from build123d import *

# Parameters (mm, degrees)
SKETCH1_R           = 5
BOSS_EXTRUDE1_DEPTH = 3
BOSS_EXTRUDE2_DEPTH = 3
BOSS_EXTRUDE3_DEPTH = 2.5
SKETCH4_R           = 3
CUT_EXTRUDE1_DEPTH  = 1
SKETCH5_R           = 1.25
CUT_EXTRUDE2_DEPTH  = 36.707142143
CUT_EXTRUDE3_DEPTH  = 3
SKETCH7_R           = 1
CUT_EXTRUDE4_DEPTH  = 36.860842154


with BuildPart() as part:
    # Sketch1 → Boss-Extrude1 (new body)
    with BuildSketch(Plane(origin=(0, 0, 0), x_dir=(1, 0, 0), z_dir=(0, 1, 0))):
        with Locations(Location((0, 0, 0), (0, 0, 270))):
            Circle(SKETCH1_R)
    extrude(amount=BOSS_EXTRUDE1_DEPTH)

    # Sketch2 → Boss-Extrude2 (add)
    with BuildSketch(Plane.XZ):
        with BuildLine():
            Line((-19, 6), (19, 6))
            ThreePointArc((19, 6), (25, 0), (19, -6))
            Line((19, -6), (-19, -6))
            ThreePointArc((-19, -6), (-25, 0), (-19, 6))
        make_face()
    extrude(amount=BOSS_EXTRUDE2_DEPTH)

    # Sketch3 → Boss-Extrude3 (add)
    with BuildSketch(Plane.XZ.offset(3)):
        with BuildLine():
            Line((-6, -19), (-6, 19))
            ThreePointArc((-6, 19), (0, 25), (6, 19))
            Line((6, 19), (6, -19))
            ThreePointArc((6, -19), (0, -25), (-6, -19))
        make_face()
    extrude(amount=-BOSS_EXTRUDE3_DEPTH)

    # Sketch4 → Cut-Extrude1 (cut)
    with BuildSketch(Plane.XZ.offset(3)):
        with Locations(Location((0, 0, 0), (0, 0, 270))):
            Circle(SKETCH4_R)
    extrude(amount=-CUT_EXTRUDE1_DEPTH, mode=Mode.SUBTRACT)

    # Sketch5 → Cut-Extrude2 (cut, through all)
    with BuildSketch(Plane.XZ.offset(2)):
        with Locations(Location((0, 0, 0), (0, 0, 270))):
            Circle(SKETCH5_R)
    extrude(amount=-CUT_EXTRUDE2_DEPTH, mode=Mode.SUBTRACT)

    # Sketch6 → Cut-Extrude3 (cut)
    with BuildSketch(Plane(origin=(0, 3, 0), x_dir=(1, 0, 0), z_dir=(0, 1, 0))):
        with BuildLine():
            Line((0.25, 2.25), (0.25, 1.984313483))
            ThreePointArc((0.25, 1.984313483), (0.367499036, 1.965946199), (0.483698652, 1.940627634))
            Line((0.483698652, 1.940627634), (0.579675692, 2.188372933))
            ThreePointArc((0.579675692, 2.188372933), (0.903104165, 2.331180574), (1.045911806, 2.0077521))
            Line((1.045911806, 2.0077521), (0.949934766, 1.760006801))
            ThreePointArc((0.949934766, 1.760006801), (1.052864326, 1.700434271), (1.15207112, 1.63484927))
            Line((1.15207112, 1.63484927), (1.331062969, 1.831193975))
            ThreePointArc((1.331062969, 1.831193975), (1.684239109, 1.847522293), (1.700567428, 1.494346153))
            Line((1.700567428, 1.494346153), (1.521575579, 1.298001448))
            ThreePointArc((1.521575579, 1.298001448), (1.596034455, 1.205269273), (1.66485, 1.108275452))
            Line((1.66485, 1.108275452), (1.902682817, 1.226702123))
            ThreePointArc((1.902682817, 1.226702123), (2.237908228, 1.114345889), (2.125551994, 0.779120478))
            Line((2.125551994, 0.779120478), (1.887719178, 0.660693807))
            ThreePointArc((1.887719178, 0.660693807), (1.923651286, 0.54732598), (1.952781662, 0.432022894))
            Line((1.952781662, 0.432022894), (2.217334807, 0.456537353))
            ThreePointArc((2.217334807, 0.456537353), (2.489335441, 0.230670899), (2.263468987, -0.041329735))
            Line((2.263468987, -0.041329735), (1.998915842, -0.065844194))
            ThreePointArc((1.998915842, -0.065844194), (1.991468353, -0.184536719), (1.97697934, -0.30257675))
            Line((1.97697934, -0.30257675), (2.232523445, -0.375285317))
            ThreePointArc((2.232523445, -0.375285317), (2.404564108, -0.684157475), (2.09569195, -0.856198138))
            Line((2.09569195, -0.856198138), (1.840147845, -0.783489572))
            ThreePointArc((1.840147845, -0.783489572), (1.790326583, -0.891476712), (1.734175003, -0.996311728))
            Line((1.734175003, -0.996311728), (1.94619742, -1.156423625))
            ThreePointArc((1.94619742, -1.156423625), (1.995043068, -1.506586591), (1.644880102, -1.555432239))
            Line((1.644880102, -1.555432239), (1.432857685, -1.395320341))
            ThreePointArc((1.432857685, -1.395320341), (1.347391287, -1.478017834), (1.257160723, -1.555489285))
            Line((1.257160723, -1.555489285), (1.39702665, -1.781380515))
            ThreePointArc((1.39702665, -1.781380515), (1.316080407, -2.125542839), (0.971918083, -2.044596596))
            Line((0.971918083, -2.044596596), (0.832052155, -1.818705367))
            ThreePointArc((0.832052155, -1.818705367), (0.722483332, -1.864944459), (0.610359921, -1.904589396))
            Line((0.610359921, -1.904589396), (0.65917969, -2.165752095))
            ThreePointArc((0.65917969, -2.165752095), (0.459373795, -2.457432749), (0.16769314, -2.257626854))
            Line((0.16769314, -2.257626854), (0.118873371, -1.996464155))
            ThreePointArc((0.118873371, -1.996464155), (0, -2), (-0.118873371, -1.996464155))
            Line((-0.118873371, -1.996464155), (-0.16769314, -2.257626854))
            ThreePointArc((-0.16769314, -2.257626854), (-0.459373795, -2.457432749), (-0.65917969, -2.165752095))
            Line((-0.65917969, -2.165752095), (-0.610359921, -1.904589396))
            ThreePointArc((-0.610359921, -1.904589396), (-0.722483332, -1.864944459), (-0.832052155, -1.818705367))
            Line((-0.832052155, -1.818705367), (-0.971918083, -2.044596596))
            ThreePointArc((-0.971918083, -2.044596596), (-1.316080407, -2.125542839), (-1.39702665, -1.781380515))
            Line((-1.39702665, -1.781380515), (-1.257160723, -1.555489285))
            ThreePointArc((-1.257160723, -1.555489285), (-1.347391287, -1.478017834), (-1.432857685, -1.395320341))
            Line((-1.432857685, -1.395320341), (-1.644880102, -1.555432239))
            ThreePointArc((-1.644880102, -1.555432239), (-1.995043068, -1.506586591), (-1.94619742, -1.156423625))
            Line((-1.94619742, -1.156423625), (-1.734175003, -0.996311728))
            ThreePointArc((-1.734175003, -0.996311728), (-1.790326583, -0.891476712), (-1.840147845, -0.783489572))
            Line((-1.840147845, -0.783489572), (-2.09569195, -0.856198138))
            ThreePointArc((-2.09569195, -0.856198138), (-2.404564108, -0.684157475), (-2.232523445, -0.375285317))
            Line((-2.232523445, -0.375285317), (-1.97697934, -0.30257675))
            ThreePointArc((-1.97697934, -0.30257675), (-1.991468353, -0.184536719), (-1.998915842, -0.065844194))
            Line((-1.998915842, -0.065844194), (-2.263468987, -0.041329735))
            ThreePointArc((-2.263468987, -0.041329735), (-2.489335441, 0.230670899), (-2.217334807, 0.456537353))
            Line((-2.217334807, 0.456537353), (-1.952781662, 0.432022894))
            ThreePointArc((-1.952781662, 0.432022894), (-1.923651286, 0.54732598), (-1.887719178, 0.660693807))
            Line((-1.887719178, 0.660693807), (-2.125551994, 0.779120478))
            ThreePointArc((-2.125551994, 0.779120478), (-2.237908228, 1.114345889), (-1.902682817, 1.226702123))
            Line((-1.902682817, 1.226702123), (-1.66485, 1.108275452))
            ThreePointArc((-1.66485, 1.108275452), (-1.596034455, 1.205269273), (-1.521575579, 1.298001448))
            Line((-1.521575579, 1.298001448), (-1.700567428, 1.494346153))
            ThreePointArc((-1.700567428, 1.494346153), (-1.684239109, 1.847522293), (-1.331062969, 1.831193975))
            Line((-1.331062969, 1.831193975), (-1.15207112, 1.63484927))
            ThreePointArc((-1.15207112, 1.63484927), (-1.052864326, 1.700434271), (-0.949934766, 1.760006801))
            Line((-0.949934766, 1.760006801), (-1.045911806, 2.0077521))
            ThreePointArc((-1.045911806, 2.0077521), (-0.903104165, 2.331180574), (-0.579675692, 2.188372933))
            Line((-0.579675692, 2.188372933), (-0.483698652, 1.940627634))
            ThreePointArc((-0.483698652, 1.940627634), (-0.367499036, 1.965946199), (-0.25, 1.984313483))
            Line((-0.25, 1.984313483), (-0.25, 2.25))
            ThreePointArc((-0.25, 2.25), (0, 2.5), (0.25, 2.25))
        make_face()
    extrude(amount=-CUT_EXTRUDE3_DEPTH, mode=Mode.SUBTRACT)

    # Sketch7 → Cut-Extrude4 (cut, through all)
    with BuildSketch(Plane.XZ.offset(3)):
        with Locations(Location((0, 23, 0), (0, 0, 270))):
            Circle(SKETCH7_R)
        with Locations(Location((0, 20, 0), (0, 0, 270))):
            Circle(SKETCH7_R)
        with Locations(Location((0, 17, 0), (0, 0, 270))):
            Circle(SKETCH7_R)
        with Locations(Location((0, 14, 0), (0, 0, 270))):
            Circle(SKETCH7_R)
        with Locations(Location((23, 0, 0), (0, 0, 270))):
            Circle(SKETCH7_R)
        with Locations(Location((20, 0, 0), (0, 0, 270))):
            Circle(SKETCH7_R)
        with Locations(Location((17, 0, 0), (0, 0, 270))):
            Circle(SKETCH7_R)
        with Locations(Location((14, 0, 0), (0, 0, 270))):
            Circle(SKETCH7_R)
        with Locations(Location((0, -23, 0), (0, 0, 270))):
            Circle(SKETCH7_R)
        with Locations(Location((0, -20, 0), (0, 0, 270))):
            Circle(SKETCH7_R)
        with Locations(Location((0, -17, 0), (0, 0, 270))):
            Circle(SKETCH7_R)
        with Locations(Location((0, -14, 0), (0, 0, 270))):
            Circle(SKETCH7_R)
        with Locations(Location((-23, 0, 0), (0, 0, 270))):
            Circle(SKETCH7_R)
        with Locations(Location((-20, 0, 0), (0, 0, 270))):
            Circle(SKETCH7_R)
        with Locations(Location((-17, 0, 0), (0, 0, 270))):
            Circle(SKETCH7_R)
        with Locations(Location((-14, 0, 0), (0, 0, 270))):
            Circle(SKETCH7_R)
    extrude(amount=-CUT_EXTRUDE4_DEPTH, mode=Mode.SUBTRACT)


solid = part.part
Could you check a few things on this model? Use its own coordinates, in mm. A direction names the side the tool comes from. Give positions to 0.01 mm unless a question says otherwise; leave off trailing zeros. Order: outer loops, then holes, each group sorted by start corner. A loop starts at its lowest first (then second) coordinate and runs counter-clockwise, first axis right, second up. Notation, with made-up numbers: (-27, 43) - (5, 43) arc R23 cw to (5, 76) - close; hole circle Ø7 at (6.5, 4.5). An arc over 180 degrees is marked (long way). One line per item, written item: value. Start each with the question number.
1. For faces 4 (the face through (0.9, -2.51, -2.86)), 5 (the face through (-15, -2, 0)), 6 (the face through (-1, 0, -1)), which set-ups out of +Z, -Z, +X, -X, +Y, -Y let a thin tool reach every point of the face, with its end or its side?
2. If I drill on probe 1 along X at (y, z) = (-1.35, 14); probe 2 along Z at (x, y) = (4.5, 1.65); probe 3 along X at (y, z) = (-1.85, -12), over which ranges is the centre line in solid material (lowest first)?
3. Imagine slicing it at B-B on z = -23. List the corners of the cut face in (x, y) for me.
4. Imagine slicing it at A-A on x = -14. List the corners of the cut face in (y, z) for me.
5. For P1, Ø2.5, axis at x = -9.5, y = -1, coming from the +Z side; P2, Ø5.5, axis at x = 0, z = 0, coming from the -Y side; P3, Ø3.5, axis at x = -1, z = 12, coming from the +Y side, each with a flat end and sliding along its axis, tell me the tip position at first contact or that it passes through.
6. Imagine slicing it at C-C on x = 10.5. List the corners of the cut face in (y, z) for me.
7. Thinking about a two-plate mould opening in Z: for faces 1 (the face through (0, -2, -19)), 2 (the face through (-5, -3, 0)), 3 (the face through (25, -1, 0)), which applies, +Z half, -Z half, draft (parallel to the pull), parting line (faces both ways), or undercut?
Values:
1. face 4: -Y
1. face 5: +Y, -Y
1. face 6: +Y
2. probe 1: -6 to -1, 1 to 6
2. probe 2: -2.18 to 2.18
2. probe 3: -6 to 6
3. outline: (-4.47, -3) - (-1, -3) - (-1, -0.5) - (-4.47, -0.5) - close; (1, -3) - (4.47, -3) - (4.47, -0.5) - (1, -0.5) - close
4. outline: (-3, -6) - (0, -6) - (0, -1) - (-3, -1) - close; (-3, 1) - (0, 1) - (0, 6) - (-3, 6) - close
5. P1: z = 6
5. P2: y = -2
5. P3: y = -0.5
6. outline: (-3, -6) - (0, -6) - (0, 6) - (-3, 6) - close
7. face 1: undercut
7. face 2: draft
7. face 3: parting line
